from build123d import *

# Parameters (mm, degrees)
F1_DEPTH = 2.8702


with BuildPart() as f1:
    # F0 (on Front) → F1 (new body, symmetric)
    with BuildSketch(Plane.XZ):
        with BuildLine():
            ThreePointArc((5.7785, 0), (5.7740449859, 0.2268628454), (5.760686813, 0.4533758847))
            ThreePointArc((5.760686813, 0.4533758847), (5.4407027929, 0.736461757), (5.0174567702, 0.7946870824))
            Line((5.0174567702, 0.7946870824), (4.1017709097, 0.6496566899))
            ThreePointArc((4.1017709097, 0.6496566899), (4.0381550424, 0.9694752516), (3.9496426065, 1.2833166759))
            Line((3.9496426065, 1.2833166759), (1.8872527745, 0.6132055982))
            ThreePointArc((1.8872527745, 0.6132055982), (1.9599440509, 0.3104246416), (1.984375, 0))
            Line((1.984375, 0), (5.7785, 0))
        make_face()
        with BuildLine():
            ThreePointArc((5.760686813, -0.4533758847), (5.7740449859, -0.2268628454), (5.7785, 0))
            Line((5.7785, 0), (1.984375, 0))
            ThreePointArc((1.984375, 0), (-1.9599440509, -0.3104246416), (1.8872527745, 0.6132055982))
            Line((1.8872527745, 0.6132055982), (3.9496426065, 1.2833166759))
            ThreePointArc((3.9496426065, 1.2833166759), (3.8367793106, 1.5892460263), (3.7002609943, 1.8853771464))
            Line((3.7002609943, 1.8853771464), (4.5263131429, 2.3062717387))
            ThreePointArc((4.5263131429, 2.3062717387), (4.8345023804, 2.6021547867), (4.9269811897, 3.0192579562))
            ThreePointArc((4.9269811897, 3.0192579562), (4.8046471547, 3.2103625915), (4.674904702, 3.3965170804))
            ThreePointArc((4.674904702, 3.3965170804), (4.5379538851, 3.5774343861), (4.3940058722, 3.7528355473))
            ThreePointArc((4.3940058722, 3.7528355473), (3.9687396612, 3.7937749409), (3.5921024484, 3.5921024484))
            Line((3.5921024484, 3.5921024484), (2.9365437516, 2.9365437516))
            ThreePointArc((2.9365437516, 2.9365437516), (2.6970927999, 3.1578899345), (2.4410133742, 3.3597666759))
            ThreePointArc((2.4410133742, 3.3597666759), (2.1698842894, 3.5409293385), (1.8853771464, 3.7002609943))
            Line((1.8853771464, 3.7002609943), (2.3062717387, 4.5263131429))
            ThreePointArc((2.3062717387, 4.5263131429), (2.3816863773, 4.9468366458), (2.2113362139, 5.3386378786))
            ThreePointArc((2.2113362139, 5.3386378786), (2.0000374143, 5.4213386346), (1.785654702, 5.4956800794))
            ThreePointArc((1.785654702, 5.4956800794), (1.5685186395, 5.5615475838), (1.348964035, 5.618839585))
            ThreePointArc((1.348964035, 5.618839585), (0.9808528714, 5.401995043), (0.7946870824, 5.0174567702))
            Line((0.7946870824, 5.0174567702), (0.6496566899, 4.1017709097))
            ThreePointArc((0.6496566899, 4.1017709097), (0.3258327786, 4.1400979953), (0, 4.1529))
            ThreePointArc((0, 4.1529), (-0.3258327786, 4.1400979953), (-0.6496566899, 4.1017709097))
            Line((-0.6496566899, 4.1017709097), (-0.7946870824, 5.0174567702))
            ThreePointArc((-0.7946870824, 5.0174567702), (-0.9808528714, 5.401995043), (-1.348964035, 5.618839585))
            ThreePointArc((-1.348964035, 5.618839585), (-1.5685186395, 5.5615475838), (-1.785654702, 5.4956800794))
            ThreePointArc((-1.785654702, 5.4956800794), (-2.0000374143, 5.4213386346), (-2.2113362139, 5.3386378786))
            ThreePointArc((-2.2113362139, 5.3386378786), (-2.3816863773, 4.9468366458), (-2.3062717387, 4.5263131429))
            Line((-2.3062717387, 4.5263131429), (-1.8853771464, 3.7002609943))
            ThreePointArc((-1.8853771464, 3.7002609943), (-2.1698842894, 3.5409293385), (-2.4410133742, 3.3597666759))
            ThreePointArc((-2.4410133742, 3.3597666759), (-2.6970927999, 3.1578899345), (-2.9365437516, 2.9365437516))
            Line((-2.9365437516, 2.9365437516), (-3.5921024484, 3.5921024484))
            ThreePointArc((-3.5921024484, 3.5921024484), (-3.9687396612, 3.7937749409), (-4.3940058722, 3.7528355473))
            ThreePointArc((-4.3940058722, 3.7528355473), (-4.5379538851, 3.5774343861), (-4.674904702, 3.3965170804))
            ThreePointArc((-4.674904702, 3.3965170804), (-4.8046471547, 3.2103625915), (-4.9269811897, 3.0192579562))
            ThreePointArc((-4.9269811897, 3.0192579562), (-4.8345023804, 2.6021547867), (-4.5263131429, 2.3062717387))
            Line((-4.5263131429, 2.3062717387), (-3.7002609943, 1.8853771464))
            ThreePointArc((-3.7002609943, 1.8853771464), (-3.8367793106, 1.5892460263), (-3.9496426065, 1.2833166759))
            ThreePointArc((-3.9496426065, 1.2833166759), (-4.0381550424, 0.9694752516), (-4.1017709097, 0.6496566899))
            Line((-4.1017709097, 0.6496566899), (-5.0174567702, 0.7946870824))
            ThreePointArc((-5.0174567702, 0.7946870824), (-5.4407027929, 0.736461757), (-5.760686813, 0.4533758847))
            ThreePointArc((-5.760686813, 0.4533758847), (-5.7740449859, 0.2268628454), (-5.7785, 0))
            ThreePointArc((-5.7785, 0), (-5.7740449859, -0.2268628454), (-5.760686813, -0.4533758847))
            ThreePointArc((-5.760686813, -0.4533758847), (-5.4407027929, -0.736461757), (-5.0174567702, -0.7946870824))
            Line((-5.0174567702, -0.7946870824), (-4.1017709097, -0.6496566899))
            ThreePointArc((-4.1017709097, -0.6496566899), (-4.0381550424, -0.9694752516), (-3.9496426065, -1.2833166759))
            ThreePointArc((-3.9496426065, -1.2833166759), (-3.8367793106, -1.5892460263), (-3.7002609943, -1.8853771464))
            Line((-3.7002609943, -1.8853771464), (-4.5263131429, -2.3062717387))
            ThreePointArc((-4.5263131429, -2.3062717387), (-4.8345023804, -2.6021547867), (-4.9269811897, -3.0192579562))
            ThreePointArc((-4.9269811897, -3.0192579562), (-4.8046471547, -3.2103625915), (-4.674904702, -3.3965170804))
            ThreePointArc((-4.674904702, -3.3965170804), (-4.5379538851, -3.5774343861), (-4.3940058722, -3.7528355473))
            ThreePointArc((-4.3940058722, -3.7528355473), (-3.9687396612, -3.7937749409), (-3.5921024484, -3.5921024484))
            Line((-3.5921024484, -3.5921024484), (-2.9365437516, -2.9365437516))
            ThreePointArc((-2.9365437516, -2.9365437516), (-2.6970927999, -3.1578899345), (-2.4410133742, -3.3597666759))
            ThreePointArc((-2.4410133742, -3.3597666759), (-2.1698842894, -3.5409293385), (-1.8853771464, -3.7002609943))
            Line((-1.8853771464, -3.7002609943), (-2.3062717387, -4.5263131429))
            ThreePointArc((-2.3062717387, -4.5263131429), (-2.3816863773, -4.9468366458), (-2.2113362139, -5.3386378786))
            ThreePointArc((-2.2113362139, -5.3386378786), (-2.0000374143, -5.4213386346), (-1.785654702, -5.4956800794))
            ThreePointArc((-1.785654702, -5.4956800794), (-1.5685186395, -5.5615475838), (-1.348964035, -5.618839585))
            ThreePointArc((-1.348964035, -5.618839585), (-0.9808528714, -5.401995043), (-0.7946870824, -5.0174567702))
            Line((-0.7946870824, -5.0174567702), (-0.6496566899, -4.1017709097))
            ThreePointArc((-0.6496566899, -4.1017709097), (-0.3258327786, -4.1400979953), (0, -4.1529))
            ThreePointArc((0, -4.1529), (0.3258327786, -4.1400979953), (0.6496566899, -4.1017709097))
            Line((0.6496566899, -4.1017709097), (0.7946870824, -5.0174567702))
            ThreePointArc((0.7946870824, -5.0174567702), (0.9808528714, -5.401995043), (1.348964035, -5.618839585))
            ThreePointArc((1.348964035, -5.618839585), (1.5685186395, -5.5615475838), (1.785654702, -5.4956800794))
            ThreePointArc((1.785654702, -5.4956800794), (2.0000374143, -5.4213386346), (2.2113362139, -5.3386378786))
            ThreePointArc((2.2113362139, -5.3386378786), (2.3816863773, -4.9468366458), (2.3062717387, -4.5263131429))
            Line((2.3062717387, -4.5263131429), (1.8853771464, -3.7002609943))
            ThreePointArc((1.8853771464, -3.7002609943), (2.1698842894, -3.5409293385), (2.4410133742, -3.3597666759))
            ThreePointArc((2.4410133742, -3.3597666759), (2.6970927999, -3.1578899345), (2.9365437516, -2.9365437516))
            Line((2.9365437516, -2.9365437516), (3.5921024484, -3.5921024484))
            ThreePointArc((3.5921024484, -3.5921024484), (3.9687396612, -3.7937749409), (4.3940058722, -3.7528355473))
            ThreePointArc((4.3940058722, -3.7528355473), (4.5379538851, -3.5774343861), (4.674904702, -3.3965170804))
            ThreePointArc((4.674904702, -3.3965170804), (4.8046471547, -3.2103625915), (4.9269811897, -3.0192579562))
            ThreePointArc((4.9269811897, -3.0192579562), (4.8345023804, -2.6021547867), (4.5263131429, -2.3062717387))
            Line((4.5263131429, -2.3062717387), (3.7002609943, -1.8853771464))
            ThreePointArc((3.7002609943, -1.8853771464), (3.8367793106, -1.5892460263), (3.9496426065, -1.2833166759))
            ThreePointArc((3.9496426065, -1.2833166759), (4.0381550424, -0.9694752516), (4.1017709097, -0.6496566899))
            Line((4.1017709097, -0.6496566899), (5.0174567702, -0.7946870824))
            ThreePointArc((5.0174567702, -0.7946870824), (5.4407027929, -0.736461757), (5.760686813, -0.4533758847))
        make_face()
    extrude(amount=F1_DEPTH, both=True)


solid = f1.part
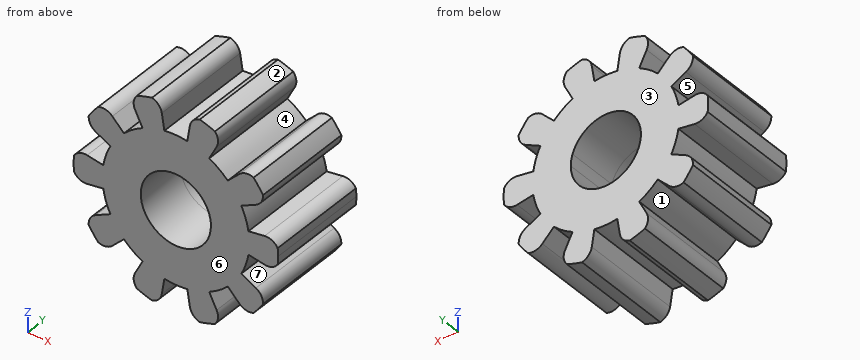
Part model, mm, in its own coordinate system. Face numbers are marked on the shaded views. A direction names the side the tool comes from. Give positions to 0.01 mm unless a question says otherwise; leave off trailing zeros. Loops run counter-clockwise (first coordinate to the right, second up) from the corner with the lowest first, then second, coordinate; pieces in that order, holes last. Notation, with made-up numbers: M 67,54.5 L 123,54.5 A25 ccw 123,87.5 Z; hole C 8,2 d6. An arc over 180 degrees is marked long. Put each result on its own line as item: value. Start each with the question number.
1) 3-axis set-ups, long thin cutter, end or side, ignore diameter. For the marked faces 5, 6 and 7: which of +Z, -Z, +X, -X, +Y, -Y reach the whole face in a straight line?
2) Pull direction X, two halves, no side cores. Call the marked faces 1, 2, 3 and 4: +X half, -X half, draft (parallel to the pull), parting line (faces both ways), or undercut.
3) Saw through at B-B (x = -3.25). List the corners of the cut face in (y, z), then the cut area to 3 significant figures.
4) Probe probe 1 along X at (y, z) = (1.7, -3.5); probe 2 along Z at (x, y) = (2.25, -2.35); probe 3 along Z at (x, y) = (-1, 0.35). List the from-to ranges inside material, lowest first.
5) Saw through at A-A (x = 0). List the corners of the cut face in (y, z).
Numbers:
1. face 5: -X, +Y, -Y
1. face 6: +Z, -Z, +X, -X, -Y
1. face 7: +X, +Y, -Y
2. face 1: undercut
2. face 2: +X half
2. face 3: draft
2. face 4: undercut
3. outline: M -2.87,-3.25 L 2.87,-3.25 L 2.87,3.25 L -2.87,3.25 Z
3. area: 37.3 mm^2
4. probe 1: -4.6 to -3.5, -2.24 to 2.24, 3.5 to 4.6
4. probe 2: -5.29 to -4.42, -3.49 to 3.49, 4.42 to 5.29
4. probe 3: -5.42 to -1.71, 1.71 to 5.42
5. outline: M -2.87,-4.15 L 2.87,-4.15 L 2.87,-1.98 L -2.87,-1.98 Z; M -2.87,1.98 L 2.87,1.98 L 2.87,4.15 L -2.87,4.15 Z
